```python
from build123d import *

# Parameters (mm, degrees)
BOSS_EXTRUDE1_DEPTH       = 55
SHELL1_T                  = -2
BOSS_EXTRUDE2_DEPTH       = 10
M3X0_5_TAPPED_HOLE1_D     = 2.5
M3X0_5_TAPPED_HOLE1_DEPTH = 7.5
M3X0_5_TAPPED_HOLE1_TIP   = 0.751075774
BOSS_EXTRUDE3_REACH       = 79.136
SKETCH5_W                 = 86
SKETCH5_H                 = 2
SKETCH6_W                 = 40
SKETCH6_H                 = 15
CUT_EXTRUDE1_DEPTH        = 10
F_3_0MM_DOWEL_HOLE1_D     = 3
F_3_0MM_DOWEL_HOLE1_DEPTH = 4
F_3_0MM_DOWEL_HOLE1_TIP   = 0.901290929
SKETCH9_W                 = 20
SKETCH9_H                 = 16
CUT_EXTRUDE2_DEPTH        = 2
FILLET1_R                 = 2


with BuildPart() as part:
    # Sketch1 → Boss-Extrude1 (new body)
    with BuildSketch(Plane.XY):
        with BuildLine():
            Line((-25, 30), (25, 30))
            ThreePointArc((25, 30), (39.142135624, 24.142135624), (45, 10))
            Line((45, 10), (45, -20))
            ThreePointArc((45, -20), (42.071067812, -27.071067812), (35, -30))
            Line((35, -30), (-35, -30))
            ThreePointArc((-35, -30), (-42.071067812, -27.071067812), (-45, -20))
            Line((-45, -20), (-45, 10))
            ThreePointArc((-45, 10), (-39.142135624, 24.142135624), (-25, 30))
        make_face()
    extrude(amount=BOSS_EXTRUDE1_DEPTH)

    # Shell1
    shell1_openings = [part.faces().sort_by_distance(p)[0] for p in [
        (0, -0.615524706, 0),
    ]]
    offset(amount=SHELL1_T, openings=shell1_openings, kind=Kind.INTERSECTION)

    # Sketch2 → Boss-Extrude2 (add)
    with BuildSketch(Plane(origin=(0, 0, 0), x_dir=(-1, 0, 0), z_dir=(0, 0, -1))):
        with BuildLine():
            Line((-23, 18.48), (-40.87732975, 18.48))
            ThreePointArc((-40.87732975, 18.48), (-34.256349172, 25.437616396), (-25, 28))
            Line((-25, 28), (-23, 28))
            Line((-23, 28), (-23, 18.48))
        make_face()
        with BuildLine():
            Line((23, 18.48), (40.87732975, 18.48))
            ThreePointArc((40.87732975, 18.48), (34.256349172, 25.437616396), (25, 28))
            Line((25, 28), (23, 28))
            Line((23, 28), (23, 18.48))
        make_face()
    extrude(amount=-BOSS_EXTRUDE2_DEPTH)

    # M3x0.5 Tapped Hole1
    with Locations(Plane(origin=(0, 0, 0), x_dir=(-1, 0, 0), z_dir=(0, 0, -1))):
        with Locations((-28.5, 22), (28.5, 22)):
            Hole(M3X0_5_TAPPED_HOLE1_D / 2, depth=M3X0_5_TAPPED_HOLE1_DEPTH)
            with Locations((0, 0, -(M3X0_5_TAPPED_HOLE1_DEPTH + M3X0_5_TAPPED_HOLE1_TIP / 2))):  # 118° drill point
                Cone(0, M3X0_5_TAPPED_HOLE1_D / 2, M3X0_5_TAPPED_HOLE1_TIP, mode=Mode.SUBTRACT)

    # Sketch5 → Boss-Extrude3 (add, up to next)
    with BuildSketch(Plane(origin=(0, 0, 0), x_dir=(-1, 0, 0), z_dir=(0, 0, -1)), mode=Mode.PRIVATE) as boss_extrude3_sk1:
        with Locations((0, -6)):
            Rectangle(SKETCH5_W, SKETCH5_H)
    boss_extrude3_tool1 = extrude(boss_extrude3_sk1.sketch, amount=-BOSS_EXTRUDE3_REACH, mode=Mode.PRIVATE) - part.part
    add(boss_extrude3_tool1.solids().sort_by_distance((0, -6, 0))[0])

    # Sketch6 → Cut-Extrude1 (cut)
    with BuildSketch(Plane(origin=(0, 0, 53), x_dir=(-1, 0, 0), z_dir=(0, 0, -1))):
        with Locations((0, 2.5)):
            Rectangle(SKETCH6_W, SKETCH6_H)
    extrude(amount=-CUT_EXTRUDE1_DEPTH, mode=Mode.SUBTRACT)

    # Ø3.0mm Dowel Hole1
    with Locations(Plane(origin=(0, -5, 0), x_dir=(1, 0, 0), z_dir=(0, 1, 0))):
        with Locations((-17, -47), (-17, -22), (17, -34.5)):
            Hole(F_3_0MM_DOWEL_HOLE1_D / 2, depth=F_3_0MM_DOWEL_HOLE1_DEPTH)
            with Locations((0, 0, -(F_3_0MM_DOWEL_HOLE1_DEPTH + F_3_0MM_DOWEL_HOLE1_TIP / 2))):  # 118° drill point
                Cone(0, F_3_0MM_DOWEL_HOLE1_D / 2, F_3_0MM_DOWEL_HOLE1_TIP, mode=Mode.SUBTRACT)

    # Sketch9 → Cut-Extrude2 (cut)
    with BuildSketch(Plane(origin=(0, -5, 0), x_dir=(1, 0, 0), z_dir=(0, 1, 0))):
        with Locations((-33, -34.5)):
            Rectangle(SKETCH9_W, SKETCH9_H)
    extrude(amount=-CUT_EXTRUDE2_DEPTH, mode=Mode.SUBTRACT)

    # Fillet1
    fillet1_edges = [part.edges().sort_by_distance(p)[0] for p in [
        (39.142135624, 24.142135624, 55),
        (0, 30, 55),
        (-39.142135624, 24.142135624, 55),
        (-45, -5, 55),
        (-42.071067812, -27.071067812, 55),
        (0, -30, 55),
        (42.071067812, -27.071067812, 55),
        (45, -5, 55),
    ]]
    fillet(fillet1_edges, radius=FILLET1_R)


solid = part.part
```
Verification items for the finished model (mm, model axes). A direction names the side the tool comes from. Round coordinates to 2 decimals unless told otherwise and drop trailing zeros. Order: outer loops, then holes, each group sorted by start corner. A loop starts at its lowest first (then second) coordinate and runs counter-clockwise, first axis right, second up. Notation, with made-up numbers: (-13.5, -13) - (37.5, -13) arc R21 cw to (37.5, 0) - close; hole circle Ø1 at (-39.5, 27.5). An arc over 180 degrees is marked (long way). Use CSV: the item, a comma, the result in double quotes. Start each with the question number.
1) Section check C-C, the plane x = 17. Record the cut outline in (y, z).
2) Section check A-A, the plane y = 4. Record the cut outline in (x, z).
3) Thickness scan on L1, parallel to Y at x = 24.5, z = 42.5; L2, parallel to X at y = 22, z = 5.5; L3, parallel to X at y = -6, z = 47. Record the ranges inside material, lowest first.
4) Section check B-B, the plane z = 24.5. Record the cut outline in (x, y).
5) Access from +Z, -Z, +X, -X, +Y, -Y to the whole of each face (thin tool, end or side, straight path). Record for faces 1 (the flat face through (-20, 2, 54)), 2 (the flat face through (-23, -6, 35)), 3 (the flat face through (43, -13, 26)).
6) Mould release check, pull along Z, two halves, no side actions. Record for faces 4 (the cylindrical face through (18.2, -6, 35.4)), 5 (the flat face through (1, -7, 26)), 6 (the conical face through (28.3, 21.92, 8.12)), 7 (the flat face through (-33, -6, 26.5)): +Z half, -Z half, draft (parallel to the pull), parting line (faces both ways), or undercut.
7) Go/stop test with flat-tipped pins: P1, Ø1.5, axis at y = -23, z = 21.5, coming from the -X side; P2, Ø7.5, axis at y = 24.5, z = 7, coming from the -X side; P3, Ø1, axis at x = -10, y = 16, coming from the -Z side. Record where each tip stops, or that it passes through.
8) Section check D-D, the plane x = -17. Record the cut outline in (y, z), plus the area to 3 significant figures.
Answers:
1,outline,"(-30, 0) - (-28, 0) - (-28, 53) - (-7, 53) - (-7, 36) - (-5, 36) - (-5, 55) - (-28, 55) arc R2 ccw to (-30, 53) - close; (-7, 0) - (-5, 0) - (-5, 33) - (-7, 33) - close; (10, 53) - (28, 53) - (28, 0) - (30, 0) - (30, 53) arc R2 ccw to (28, 55) - (10, 55) - close"
2,outline,"(-45, 0) - (-43, 0) - (-43, 53) - (-20, 53) - (-20, 55) - (-43, 55) arc R2 ccw to (-45, 53) - close; (20, 53) - (43, 53) - (43, 0) - (45, 0) - (45, 53) arc R2 ccw to (43, 55) - (20, 55) - close"
3,L1,"y = -30 to -28, -7 to -5, 28 to 30"
3,L2,"x = -41 to -29.75, -27.25 to -23, 23 to 27.25, 29.75 to 41"
3,L3,"x = -45 to -18.5, -15.5 to 45"
4,outline,"(-45, -20) arc R10 ccw to (-35, -30) - (35, -30) arc R10 ccw to (45, -20) - (45, 10) arc R20 ccw to (25, 30) - (-25, 30) arc R20 ccw to (-45, 10) - close; hole (-43, -20) arc R8 ccw to (-35, -28) - (35, -28) arc R8 ccw to (43, -20) - (43, -7) - (-43, -7) - close; hole (-43, -5) - (43, -5) - (43, 10) arc R18 ccw to (25, 28) - (-25, 28) arc R18 ccw to (-43, 10) - close"
5,face 1,"+Z, -Z"
5,face 2,"none"
5,face 3,"-Z"
6,face 4,"undercut"
6,face 5,"draft"
6,face 6,"-Z half"
6,face 7,"undercut"
7,P1,"stops at x = -44.74"
7,P2,"stops at x = -41.87"
7,P3,"stops at z = 53"
8,outline,"(-30, 0) - (-28, 0) - (-28, 53) - (-7, 53) - (-7, 48.5) - (-5, 48.5) - (-5, 55) - (-28, 55) arc R2 ccw to (-30, 53) - close; (-7, 0) - (-5, 0) - (-5, 20.5) - (-7, 20.5) - close; (-7, 23.5) - (-5, 23.5) - (-5, 45.5) - (-7, 45.5) - close; (10, 53) - (28, 53) - (28, 0) - (30, 0) - (30, 53) arc R2 ccw to (28, 55) - (10, 55) - close"
8,area,"394 mm²"
